from build123d import *

# Parameters (mm, degrees)
SKETCH1_R           = 4.05
BOSS_EXTRUDE1_DEPTH = 4


with BuildPart() as part:
    # Sketch1 → Boss-Extrude1 (new body)
    with BuildSketch(Plane(origin=(0, 0, 0), x_dir=(1, 0, 0), z_dir=(0, 1, 0))):
        Polygon((15, -15), (-110, -15), (-110, 15), (-15, 110), (15, 110), align=None)
        with Locations((-100, 0)):
            Circle(SKETCH1_R, mode=Mode.SUBTRACT)
        with Locations((-50, 0)):
            Circle(SKETCH1_R, mode=Mode.SUBTRACT)
        Circle(SKETCH1_R, mode=Mode.SUBTRACT)
        with Locations((0, 100)):
            Circle(SKETCH1_R, mode=Mode.SUBTRACT)
        with Locations((0, 50)):
            Circle(SKETCH1_R, mode=Mode.SUBTRACT)
    extrude(amount=BOSS_EXTRUDE1_DEPTH)


solid = part.part
Read the model definition and answer for the solid it produces. Units are mm, in the model's axes. Coordinates: 2 decimals unless noted, no trailing zeros. Loops run counter-clockwise (first coordinate to the right, second up) from the corner with the lowest first, then second, coordinate; pieces in that order, holes last. Notation, with made-up numbers: (-2, -11) -> (42, -11) arc R17 cw to (42, 9) -> close; hole circle Ø9 at (5, 0). An arc over 180 degrees is marked (long way). Write item = value, one per line. Start each with the question number.
1) The part is cut by section A-A, the plane y = 1.65. Determine the outline of the cut face in (x, z), plus the area to 3 significant figures.
2) The part is cut by section C-C, the plane x = -50. Determine the outline of the cut face in (y, z), plus the area to 3 significant figures.
3) The part is cut by section D-D, the plane x = 0. Determine the outline of the cut face in (y, z).
4) The part is cut by section B-B, the plane z = -100. Determine the outline of the cut face in (x, y), plus the area to 3 significant figures.
5) The mould has two halves that part along X. Classify faces 1 (the face through (-33, 0, -34)), 2 (the face through (-110, 2, 0)), 3 (the face through (-0.527, 1.972, -54.016)): pulls with the +X half, pulls with the -X half, needs draft (parallel to the pull), parting line crosses it, or undercut.
6) Find the intervals of material crossed by L1, parallel to Z at x = 0, y = 2.9; L2, parallel to Z at x = 1.5, y = 1.15, in increasing order. Write a range as from..to.
Result:
q1.outline = (-110, -15) -> (-15, -110) -> (15, -110) -> (15, 15) -> (-110, 15) -> close; hole circle Ø8.1 at (-100, 0); hole circle Ø8.1 at (-50, 0); hole circle Ø8.1 at (0, -100); hole circle Ø8.1 at (0, -50); hole circle Ø8.1 at (0, 0)
q1.area = 10,900 mm²
q2.outline = (0, -75) -> (4, -75) -> (4, -4.05) -> (0, -4.05) -> close; (0, 4.05) -> (4, 4.05) -> (4, 15) -> (0, 15) -> close
q2.area = 328 mm²
q3.outline = (0, -110) -> (4, -110) -> (4, -104.05) -> (0, -104.05) -> close; (0, -95.95) -> (4, -95.95) -> (4, -54.05) -> (0, -54.05) -> close; (0, -45.95) -> (4, -45.95) -> (4, -4.05) -> (0, -4.05) -> close; (0, 4.05) -> (4, 4.05) -> (4, 15) -> (0, 15) -> close
q4.outline = (-25, 0) -> (-4.05, 0) -> (-4.05, 4) -> (-25, 4) -> close; (4.05, 0) -> (15, 0) -> (15, 4) -> (4.05, 4) -> close
q4.area = 128 mm²
q5.face_1 = needs draft
q5.face_2 = pulls with the -X half
q5.face_3 = undercut
q6.L1 = -110..-104.05, -95.95..-54.05, -45.95..-4.05, 4.05..15
q6.L2 = -110..-103.76, -96.24..-53.76, -46.24..-3.76, 3.76..15
